Work out the finished part from the listing and answer in its coordinate system (mm). A direction names the side the tool comes from. Give positions to 0.01 mm unless a question says otherwise; leave off trailing zeros. Loops run counter-clockwise (first coordinate to the right, second up) from the corner with the lowest first, then second, coordinate; pieces in that order, holes last. Notation, with made-up numbers: (-38, 53) - (-20, 53) arc R19 ccw to (-20, 82) - close; hole circle Ø8 at (-37, 44.5). An arc over 180 degrees is marked (long way). Use CSV: the item, a comma, the result in double quotes.
from build123d import *

# Parameters (mm, degrees)
SKETCH2_R           = 4
BOSS_EXTRUDE1_DEPTH = 0.2


with BuildPart() as part:
    # Sketch1 → Revolve1 (revolve)
    with BuildSketch(Plane.XY):
        Polygon((4, -3.284366974), (4, 9.669000537), (6.5, 9.669000537), (6.5, 14.669000537), (8.448345124, 14.669000537), (9.5, 10.692316782), (7.7, 3.192316782), (9.5, -4.307683218), (8.448345124, -8.284366974), (6.5, -8.284366974), (6.5, -3.284366974), align=None)
    revolve(axis=Axis((0, 42.323455848, 0), (0, -1, 0)))

    # Sketch2 → Boss-Extrude1 (add)
    with BuildSketch(Plane.XZ.offset(3.284366974)):
        Circle(SKETCH2_R)
    extrude(amount=-BOSS_EXTRUDE1_DEPTH)


solid = part.part
Item 1: A cutting plane is placed at D-D on y = -2. Determine the outline of the cut face in (x, z).
Determined:
outline,"circle Ø17.89 at (0, 0); hole circle Ø8 at (0, 0)"
Item 2: A cutting plane is placed at B-B on z = 0. Determine the outline of the cut face in (x, y), and give its area (3 significant figures).
Determined:
outline,"(-9.5, -4.31) - (-8.45, -8.28) - (-6.5, -8.28) - (-6.5, -3.28) - (6.5, -3.28) - (6.5, -8.28) - (8.45, -8.28) - (9.5, -4.31) - (7.7, 3.19) - (9.5, 10.69) - (8.45, 14.67) - (6.5, 14.67) - (6.5, 9.67) - (4, 9.67) - (4, -3.08) - (-4, -3.08) - (-4, 9.67) - (-6.5, 9.67) - (-6.5, 14.67) - (-8.45, 14.67) - (-9.5, 10.69) - (-7.7, 3.19) - close"
area,"169 mm²"
Item 3: The mould has two halves that part along Z. Classify faces 1 (the cylindrical face through (-5.158, 12.204, -3.955)), 2 (the flat face through (-2.5, 14.669, -6.2)), 3 (the conical face through (-1.106, -8.091, 8.427)): pulls with the +Z half, pulls with the -Z half, needs draft (parallel to the pull), parting line crosses it, or undercut.
Determined:
face 1,"undercut"
face 2,"needs draft"
face 3,"parting line crosses it"
Item 4: A cutting plane is placed at A-A on x = 0. Determine the outline of the cut face in (y, z), and give its area (3 significant figures).
Determined:
outline,"(-8.28, -8.45) - (-4.31, -9.5) - (3.19, -7.7) - (10.69, -9.5) - (14.67, -8.45) - (14.67, -6.5) - (9.67, -6.5) - (9.67, -4) - (-3.08, -4) - (-3.08, 4) - (9.67, 4) - (9.67, 6.5) - (14.67, 6.5) - (14.67, 8.45) - (10.69, 9.5) - (3.19, 7.7) - (-4.31, 9.5) - (-8.28, 8.45) - (-8.28, 6.5) - (-3.28, 6.5) - (-3.28, -6.5) - (-8.28, -6.5) - close"
area,"169 mm²"
Item 5: A cutting plane is placed at C-C on y = 4.5. Determine the outline of the cut face in (x, z), and give its area (3 significant figures).
Determined:
outline,"circle Ø16.03 at (0, 0); hole circle Ø8 at (0, 0)"
area,"151 mm²"
Item 6: Given P1, Ø4, axis at x = -1.5, z = 3, coming from the +Y side; P2, Ø2.5, axis at x = -1, z = 1, coming from the +Y side; P3, Ø8, axis at x = -4.5, y = 11.5, coming from the -Z side; P4, Ø1, axis at x = -7, z = 7.5, coming from the -Y side, each flat-ended and moving along its own axis, determine where each tip first touches the part or whether it passes through.
Determined:
P1,"stops at y = 9.67"
P2,"stops at y = -3.08"
P3,"stops at z = -9.48"
P4,"passes through"
Item 7: Find the intervals of material crossed by line 1 (Y direction, x = -1.5, z = -5.75); line 2 (Z direction, x = 0, y = -6.7); line 3 (Y direction, x = 1, z = 2.75), in increasing order.
Determined:
line 1,"y = -3.28 to 9.67"
line 2,"z = -8.87 to -6.5, 6.5 to 8.87"
line 3,"y = -3.28 to -3.08"
Item 8: For faces 4 (the conical face through (-6.5, 1.1, -5)), 5 (the cylindrical face through (-5.158, -5.749, -3.955)), 6 (the flat face through (2.5, -8.284, -6.2)), 7 (the flat face through (0, -3.084, 0)), determine the directions among +Z, -Z, +X, -X, +Y, -Y from which every point of the face is accessible in a straight line to the end or side of a thin tool.
Determined:
face 4,"none"
face 5,"-Y"
face 6,"+Z, -Z, +X, -X, -Y"
face 7,"+Y"
